```python
from build123d import *

# Parameters (mm, degrees)
SKETCH1_W           = 30
SKETCH1_H           = 30
SKETCH1_R           = 14.25
SKETCH1_R_2         = 1.5
BOSS_EXTRUDE1_DEPTH = 6.66
BOSS_EXTRUDE2_DEPTH = 1
CIRPATTERN7_COUNT   = 3
SKETCH3_R           = 2.25
CUT_EXTRUDE2_DEPTH  = 23.234108932
SKETCH4_R           = 3.25
SKETCH4_R_2         = 2.25
BOSS_EXTRUDE3_DEPTH = 4.1
FILLET1_R           = 2.5
CUT_EXTRUDE4_START  = -0.5
SKETCH6_R           = 8
SKETCH6_R_2         = 3.25
CUT_EXTRUDE4_DEPTH  = 0.5
CUT_EXTRUDE5_DEPTH  = 5.66
FILLET4_R           = 2.5
FILLET5_R           = 2.5


with BuildPart() as part:
    # Sketch1 → Boss-Extrude1 (new body)
    with BuildSketch(Plane.XY):
        Rectangle(SKETCH1_W, SKETCH1_H)
        Circle(SKETCH1_R, mode=Mode.SUBTRACT)
        with Locations((-12.5, 12.5)):
            Circle(SKETCH1_R_2, mode=Mode.SUBTRACT)
        with Locations((12.5, 12.5)):
            Circle(SKETCH1_R_2, mode=Mode.SUBTRACT)
        with Locations((12.5, -12.5)):
            Circle(SKETCH1_R_2, mode=Mode.SUBTRACT)
        with Locations((-12.5, -12.5)):
            Circle(SKETCH1_R_2, mode=Mode.SUBTRACT)
    extrude(amount=BOSS_EXTRUDE1_DEPTH)

    # Sketch2 → Boss-Extrude2 (add)
    with BuildSketch(Plane.XY):
        with BuildLine():
            Line((-0.75, 8.968695557), (-0.75, 14.230249471))
            ThreePointArc((-0.75, 14.230249471), (-0.375130005, 14.245061512), (0, 14.25))
            Line((0, 14.25), (0, 0))
            Line((0, 0), (-12.340862004, -7.125))
            ThreePointArc((-12.340862004, -7.125), (-12.52415015, -6.797658642), (-12.698757544, -6.465605683))
            Line((-12.698757544, -6.465605683), (-8.142118191, -3.834828726))
            ThreePointArc((-8.142118191, -3.834828726), (-7.794228634, 4.5), (-0.75, 8.968695557))
        make_face()
    boss_extrude2 = extrude(amount=BOSS_EXTRUDE2_DEPTH)

    # CirPattern7: Boss-Extrude2 ×3 about axis
    cirpattern7_axis = Axis((0, 0, 0), (0, 0, 1))
    for i in range(1, CIRPATTERN7_COUNT):
        add(boss_extrude2.rotate(cirpattern7_axis, i * 360 / CIRPATTERN7_COUNT))

    # Sketch3 → Cut-Extrude2 (cut, through all)
    with BuildSketch(Plane.XY):
        with Locations(Location((0, 0, 0), (0, 0, 180))):
            Circle(SKETCH3_R)
    extrude(amount=CUT_EXTRUDE2_DEPTH, mode=Mode.SUBTRACT)

    # Sketch4 → Boss-Extrude3 (add)
    with BuildSketch(Plane.XY.offset(1)):
        with Locations(Location((0, 0, 0), (0, 0, 180))):
            Circle(SKETCH4_R)
        Circle(SKETCH4_R_2, mode=Mode.SUBTRACT)
    extrude(amount=BOSS_EXTRUDE3_DEPTH)

    # Fillet1
    fillet1_edges = [part.edges().sort_by_distance(p)[0] for p in [
        (15, -15, 3.33),
        (-15, -15, 3.33),
        (-15, 15, 3.33),
        (15, 15, 3.33),
    ]]
    fillet(fillet1_edges, radius=FILLET1_R)

    # Sketch6 → Cut-Extrude4 (cut)
    with BuildSketch(Plane.XY.offset(1).offset(CUT_EXTRUDE4_START)):
        Circle(SKETCH6_R)
        Circle(SKETCH6_R_2, mode=Mode.SUBTRACT)
    extrude(amount=CUT_EXTRUDE4_DEPTH, mode=Mode.SUBTRACT)

    # Sketch5 → Cut-Extrude5 (cut)
    with BuildSketch(Plane.XY.offset(6.66)):
        Polygon((-15, -5.283121635), (-12.5, -9.613248654), (-15, -11.056624327), align=None)
    extrude(amount=-CUT_EXTRUDE5_DEPTH, mode=Mode.SUBTRACT)

    # Fillet4
    fillet4_edges = [part.edges().sort_by_distance(p)[0] for p in [
        (-12.5, -9.613248654, 3.83),
    ]]
    fillet(fillet4_edges, radius=FILLET4_R)

    # Fillet5
    # the kernel refuses this fillet: 2.5 mm, written as the material it takes off along each edge
    with BuildSketch(Plane(origin=(-15, -11.056624327, 9.893983241), x_dir=(0, -1, 0), z_dir=(0, 0, -1))) as fillet5_piece_1:
        with BuildLine():
            CenterArc((1.293593296, -2.5), FILLET5_R, 90, 46.920482858)
            Line((-0.532422943, -0.792468245), (-0.715024567, -0.62171507))
            ThreePointArc((-0.715024567, -0.62171507), (-0.409882024, -0.209936491), (-0.216506351, 0.125))
            Line((-0.216506351, 0.125), (0, 0.25))
            Line((0, 0.25), (1.293593296, 0.25))
            Line((1.293593296, 0.25), (1.293593296, 0))
        make_face()
    extrude(amount=8.893983241, mode=Mode.SUBTRACT)
    with BuildSketch(Plane(origin=(-15, -5.283121635, 8.334682453), x_dir=(0.4999999999999945, -0.8660254037844419, 0), z_dir=(0, 0, -1))) as fillet5_piece_2:
        with BuildLine():
            CenterArc((FILLET5_R * 0.267949192431, -FILLET5_R), FILLET5_R, 90, 30)
            Line((-FILLET5_R * 0.232050807569, -FILLET5_R * 0.133974596216), (0, 0))
            Line((0, 0), (FILLET5_R * 0.267949192431, 0))
        make_face()
    extrude(amount=7.334682453, mode=Mode.SUBTRACT)


solid = part.part
```
CAD build for the part. Positions are in the model's coordinates, mm. A direction names the side the tool comes from. Coordinates: 2 decimals unless noted, no trailing zeros. Order: outer loops, then holes, each group sorted by start corner. A loop starts at its lowest first (then second) coordinate and runs counter-clockwise, first axis right, second up. Notation, with made-up numbers: (-14.75, 17.5) - (7.25, 17.5) arc R9 ccw to (7.25, 34.5) - close; hole circle Ø1 at (-4, -7). An arc over 180 degrees is marked (long way). Use a Markdown table: item, result. Add a question column.
(1) Saw through at B-B (y = 0). Give the cut face in (x, z), then the cut area to 3 significant figures.
(2) Drill centre lines: line 1 along Y through (x, z) = (0, 0.55); line 2 along Y through (x, z) = (0, 3.15); line 3 along X through (y, z) = (-3, 0.75). Where is each one in solid material? Low to high. Write a range as [from, to].
(3) Saw through at C-C (x = 0). Give the cut face in (y, z).
(4) Saw through at A-A (z = 2.25). Give the cut face in (x, y).
(5) Pull direction X, two halves, no side cores. Call faces 1 (the face through (0, 15, 3)), 2 (the face through (9.702, -6.468, 0.493)), 3 (the face through (-14.287, 14.248, 3.377)): +X half, -X half, draft (parallel to the pull), parting line (faces both ways), or undercut.
(6) Flat gauge pins, fed straight in: pin 1 (6 mm diameter, centred on x = -1.5, y = 11, fed in from +Z); pin 2 (12 mm diameter, centred on x = 11, y = 3.5, fed in from -Z); pin 3 (17.5 mm diameter, centred on x = 3, y = 1, fed in from +Z). Where does each tip first touch, or does it go through?
(7) Saw through at D-D (z = 5.5). Give the cut face in (x, y).
(8) Which spindle directions (+Z, -Z, +X, -X, +Y, -Y) get a long thin tool onto all of the face, cutting with end or side? Do faces 4 (the face through (-0.75, 11.6, 0.5)), 5 (the face through (-1.73, -7.81, 0.75)), 6 (the face through (0, -15, 3)), 7 (the face through (0, -3, 0)), 8 (the face through (-14.214, -6.645, 3.87)). Say none if no direction does.
Solved:
| question | item | result |
|---|---|---|
| 1 | outline | (-15, 0) - (-14.25, 0) - (-14.25, 6.66) - (-15, 6.66) - close; (-9, 0) - (-2.25, 0) - (-2.25, 5.1) - (-3.25, 5.1) - (-3.25, 0.5) - (-8, 0.5) - (-8, 1) - (-9, 1) - close; (2.25, 0) - (9, 0) - (9, 1) - (8, 1) - (8, 0.5) - (3.25, 0.5) - (3.25, 5.1) - (2.25, 5.1) - close; (14.25, 0) - (15, 0) - (15, 6.66) - (14.25, 6.66) - close |
| 1 | area | 26.9 mm² |
| 2 | line 1 | y = [-15, -14.25], [-9, -8], [-3.25, -2.25], [2.25, 3.25], [8, 15] |
| 2 | line 2 | y = [-15, -14.25], [-3.25, -2.25], [2.25, 3.25], [14.25, 15] |
| 2 | line 3 | x = [-15, -13.93], [-8.49, -7.42], [-1.25, 1.25], [7.42, 8.49], [13.93, 15] |
| 3 | outline | (-15, 0) - (-14.25, 0) - (-14.25, 6.66) - (-15, 6.66) - close; (-9, 0) - (-2.25, 0) - (-2.25, 5.1) - (-3.25, 5.1) - (-3.25, 0.5) - (-8, 0.5) - (-8, 1) - (-9, 1) - close; (2.25, 0) - (15, 0) - (15, 6.66) - (14.25, 6.66) - (14.25, 1) - (8, 1) - (8, 0.5) - (3.25, 0.5) - (3.25, 5.1) - (2.25, 5.1) - close |
| 4 | outline | (-15, -12.5) arc R2.5 ccw to (-12.5, -15) - (12.5, -15) arc R2.5 ccw to (15, -12.5) - (15, 12.5) arc R2.5 ccw to (12.5, 15) - (-12.5, 15) arc R2.5 ccw to (-15, 12.5) - (-15, -4.61) arc R2.5 ccw to (-14.67, -5.86) - (-13.75, -7.45) arc R2.5 cw to (-14.21, -10.52) arc R2.5 ccw to (-15, -12.35) - close; circle Ø6.5 at (0, 0); hole circle Ø28.5 at (0, 0); hole circle Ø3 at (-12.5, -12.5); hole circle Ø3 at (-12.5, 12.5); hole circle Ø4.5 at (0, 0); hole circle Ø3 at (12.5, -12.5); hole circle Ø3 at (12.5, 12.5) |
| 5 | face 1 | draft |
| 5 | face 2 | undercut |
| 5 | face 3 | -X half |
| 6 | pin 1 | stops at z = 1 |
| 6 | pin 2 | stops at z = 0 |
| 6 | pin 3 | stops at z = 5.1 |
| 7 | outline | (-15, -12.5) arc R2.5 ccw to (-12.5, -15) - (12.5, -15) arc R2.5 ccw to (15, -12.5) - (15, 12.5) arc R2.5 ccw to (12.5, 15) - (-12.5, 15) arc R2.5 ccw to (-15, 12.5) - (-15, -4.61) arc R2.5 ccw to (-14.67, -5.86) - (-13.75, -7.45) arc R2.5 cw to (-14.21, -10.52) arc R2.5 ccw to (-15, -12.35) - close; hole circle Ø28.5 at (0, 0); hole circle Ø3 at (-12.5, -12.5); hole circle Ø3 at (-12.5, 12.5); hole circle Ø3 at (12.5, -12.5); hole circle Ø3 at (12.5, 12.5) |
| 8 | face 4 | +Z, -Z |
| 8 | face 5 | +Z |
| 8 | face 6 | +Z, -Z, +X, -X, -Y |
| 8 | face 7 | -Z, +X, -X, +Y, -Y |
| 8 | face 8 | +Z, -X |
